from build123d import *

# Parameters (mm, degrees)
F0_R     = 76.2
F1_DEPTH = 25.4
F4_R     = 6.35
F5_DEPTH = 25.4
F6_T     = 5.08
F8_DEPTH = 5.081


# Not quite as in the source:
# - a shell that OpenCascade refuses in one call is made with other operations: the cavity is built on its own and cut out


with BuildPart() as f1:
    # F0 (on Front) → F1 (new body)
    with BuildSketch(Plane.XZ):
        Circle(F0_R)
    extrude(amount=F1_DEPTH)

    # F2 (on Right) → F3 (revolve, cut)
    with BuildSketch(Plane.YZ):
        Polygon((-12.7, 65.1145875454), (0, 76.22641325), (-12.7, 76.22641325), (-25.3041852266, 76.22641325), align=None)
    revolve(axis=Axis((0, -25.4, 0), (0, -1, 0)), mode=Mode.SUBTRACT)

    # F4 (on face) → F5 (cut)
    with BuildSketch(Plane.XZ.offset(25.4)):
        Circle(F4_R)
    extrude(amount=-F5_DEPTH, mode=Mode.SUBTRACT)

    # F6: shell of thickness 5.08, made by hand


with BuildPart() as f6_core1:
    # F6_t2: copy of F1
    add(f1.part)

    # the walls: a layer under each face that stays
    f6_faces = [f6_core1.faces().sort_by_distance(p)[0] for p in [
        (-76.2, -0.0150942016, 0),
        (0, -6.3650942016, -70.6572937727),
        (-6.35, -12.7, 0),
        (0, -18.9871122894, -70.6572937727),
        (-50.8, -25.4, -50.8),
        (-76.2, -25.3371122894, 0),
    ]]
    thicken(f6_faces, amount=-F6_T, mode=Mode.SUBTRACT)

    # F6_s3 → F6_t4 (revolve, cut)
    with BuildSketch(Plane.YZ):
        Polygon((-12.6998566811, 65.1909254772), (-9.3549115607, 61.2913973417), (-12.712693419, 58.3535164942), (-16.0594203306, 61.3039845692), align=None)
    revolve(axis=Axis((0, -12.7, 0), (0, -1, 0)), mode=Mode.SUBTRACT)


with BuildPart() as f1_1:
    add(f1.part)

    # what is left inside the walls is the cavity
    f6_cavity = [f6_core1.part.solids().sort_by_distance(p)[0] for p in [
        (0, -0.0508, -23.158816),
    ]]
    add(f6_cavity, mode=Mode.SUBTRACT)

    # F7 (on face) → F8 (cut, through all)
    with BuildSketch(Plane(origin=(0, -20.32, 0), x_dir=(-1, 0, 0), z_dir=(0, 1, 0))):
        with BuildLine():
            ThreePointArc((50.750755659, -15.1466698341), (52.4068897458, -7.6536732487), (52.9628247644, 0))
            ThreePointArc((52.9628247644, 0), (52.4068897458, 7.6536732487), (50.750755659, 15.1466698341))
            Line((50.750755659, 15.1466698341), (15.2094055185, 6.3428222009))
            ThreePointArc((15.2094055185, 6.3428222009), (16.1584836664, 3.2343183675), (16.4789990503, 0))
            ThreePointArc((16.4789990503, 0), (16.1584836664, -3.2343183675), (15.2094055185, -6.3428222009))
            Line((15.2094055185, -6.3428222009), (50.750755659, -15.1466698341))
        make_face()
        with BuildLine():
            ThreePointArc((-38.4927786886, -36.3781087449), (-26.4814123822, -45.8671517021), (-12.2579769704, -51.524778579))
            Line((-12.2579769704, -51.524778579), (-2.1116576016, -16.343142656))
            ThreePointArc((-2.1116576016, -16.343142656), (-8.2394995251, -14.2712318065), (-13.0977479169, -10.000320455))
            Line((-13.0977479169, -10.000320455), (-38.4927786886, -36.3781087449))
        make_face()
        with BuildLine():
            Line((-2.1116576016, 16.343142656), (-12.2579769704, 51.524778579))
            ThreePointArc((-12.2579769704, 51.524778579), (-26.4814123822, 45.8671517021), (-38.4927786886, 36.3781087449))
            Line((-38.4927786886, 36.3781087449), (-13.0977479169, 10.000320455))
            ThreePointArc((-13.0977479169, 10.000320455), (-8.2394995251, 14.2712318065), (-2.1116576016, 16.343142656))
        make_face()
    extrude(amount=-F8_DEPTH, mode=Mode.SUBTRACT)


solid = f1_1.part
Work out the finished part from the listing and answer in its coordinate system (mm). A direction names the side the tool comes from. Coordinates: 2 decimals unless noted, no trailing zeros. Write each loop counter-clockwise with the first axis right and the second up, starting at its lowest first coordinate (ties: lowest second). Pieces come first, ordered by that corner, then holes. Notation, with made-up numbers: M 45.25,55 L 80.25,55 A24 ccw 80.25,86 Z; hole C -38.75,15 d8. An arc over 180 degrees is marked long. Use one line per item in the form item = value. Start each with the question number.
1. Straight lines are drawn through the part: probe 1 along Z at (x, y) = (5.5, -17); probe 2 along Z at (x, y) = (0, -17.25); probe 3 along X at (y, z) = (-22, -3). For each, find the intervals that lie inside material, in ascending order. Write a range as from..to.
2. Each of these flat-tipped pins is pushed along its axis until it touches: P1, Ø3, axis at x = -22.5, z = -26.5, coming from the +Y side; P2, Ø4, axis at y = -12.5, z = 21.5, coming from the +X side; P3, Ø10, axis at y = -18, z = 0.5, coming from the -X side. Where does it stop, or does it pass through?
3. The mould has two halves that part along Z. Classify faces 5 (the face through (16, -25.4, 1)), 6 (the face through (39.95, -13.31, -52.1)), 7 (the face through (26.295, -22.824, 45.974)): released by +Z, released by -Z, zero draft, split by the parting line, or undercut.
4. The part is cut by section A-A (y = -2). Give the vertices of the cut face in (x, z), plus the area to 3 significant figures.
5. A tool of negligible diameter and unlimited length cuts with its end or side. For faces 1 (the face through (26, -22.8, 23.4)), 2 (the face through (10.902, -10.302, 3.433)), 3 (the face through (-65.248, -11.907, -8.567)), 4 (the face through (5, 0, -5)), from which of +Z, -Z, +X, -X, +Y, -Y can it reach the whole face along a straight path? Write none if from no direction.
Evaluation:
q1.probe_1 = -68.69..-61.89, -10.02..-3.17, 3.17..10.02, 61.89..68.69
q1.probe_2 = -69.13..-62.35, -11.43..-6.35, 6.35..11.43, 62.35..69.13
q1.probe_3 = -73.25..-52.88, -16.2..-5.6, 5.6..73.25
q2.P1 = -20.32
q2.P2 = 63.61
q2.P3 = -74.19
q3.face_5 = zero draft
q3.face_6 = split by the parting line
q3.face_7 = undercut
q4.outline = C 0,0 d148.95; C 0,0 d22.86; hole C 0,0 d135.45; hole C 0,0 d12.7
q4.area = 3,300 mm^2
q5.face_1 = +Y, -Y
q5.face_2 = +Y
q5.face_3 = none
q5.face_4 = +Z, -Z, +X, -X, +Y
